Check sheet for the modelled part. Datum: model origin and axes. Units: mm. A direction names the side the tool comes from. Coordinates: 2 decimals unless noted, no trailing zeros. Write each loop counter-clockwise with the first axis right and the second up, starting at its lowest first coordinate (ties: lowest second). Pieces come first, ordered by that corner, then holes. Notation, with made-up numbers: (-13, 27.25) -> (39, 27.25) arc R31 cw to (39, 55.25) -> close; hole circle Ø1 at (57, 52). An arc over 180 degrees is marked (long way). Put each result on its own line as item: value.
```python
from build123d import *

# Parameters (mm, degrees)
SKETCH1_R           = 2.667
BOSS_EXTRUDE1_DEPTH = 4.7625
BOSS_EXTRUDE2_DEPTH = 50.8
SKETCH4_R           = 3.302
CUT_EXTRUDE1_DEPTH  = 55.626
BOSS_EXTRUDE3_DEPTH = 50.038
CUT_EXTRUDE5_DEPTH  = 46.0375
BOSS_EXTRUDE4_DEPTH = 3.175
BOSS_EXTRUDE5_DEPTH = 3.175
FILLET1_R           = 5.08
FILLET2_R           = 5.08


with BuildPart() as part:
    # Sketch1 → Boss-Extrude1 (new body)
    with BuildSketch(Plane(origin=(0, 0, 0), x_dir=(1, 0, 0), z_dir=(0, 1, 0))):
        Polygon((37.846, 50.038), (33.907923994, 0), (0, 0), (0, 50.038), align=None)
        with Locations(Location((12.7, 37.338, 0), (0, 0, 90))):
            Circle(SKETCH1_R, mode=Mode.SUBTRACT)
        with Locations(Location((25.4, 37.338, 0), (0, 0, 90))):
            Circle(SKETCH1_R, mode=Mode.SUBTRACT)
        with Locations(Location((12.7, 11.938, 0), (0, 0, 90))):
            Circle(SKETCH1_R, mode=Mode.SUBTRACT)
        with Locations(Location((25.4, 11.938, 0), (0, 0, 90))):
            Circle(SKETCH1_R, mode=Mode.SUBTRACT)
    extrude(amount=BOSS_EXTRUDE1_DEPTH)

    # Sketch2 → Boss-Extrude2 (add)
    with BuildSketch(Plane.XZ):
        Polygon((29.2288268, -1.246852262), (33.068773405, -50.038), (37.846, -50.038), (33.907923994, 0), (29.130697399, 0), (29.160105192, -0.373661443), align=None)
    extrude(amount=-BOSS_EXTRUDE2_DEPTH)

    # Sketch4 → Cut-Extrude1 (cut)
    with BuildSketch(Plane(origin=(28.951373786, 0, 2.278522532), x_dir=(-0.07845909572784877, 0, 0.9969173337331276), z_dir=(-0.9969173337331276, 0, -0.07845909572784877))):
        with Locations((-27.304568176, 25.4)):
            Circle(SKETCH4_R)
    extrude(amount=-CUT_EXTRUDE1_DEPTH, mode=Mode.SUBTRACT)

    # Sketch5 → Boss-Extrude3 (add)
    with BuildSketch(Plane.XY):
        Polygon((2.157923994, 4.7625), (33.907923994, 16.318554938), (33.907923994, 4.7625), align=None)
    extrude(amount=-BOSS_EXTRUDE3_DEPTH)

    # Sketch7 → Cut-Extrude5 (cut)
    with BuildSketch(Plane(origin=(0, 50.8, 0), x_dir=(1, 0, 0), z_dir=(0, 1, 0))):
        Polygon((33.068773405, 50.038), (31.224674361, 26.6065), (2.157923994, 26.6065), (2.157923994, 50.038), align=None)
        Polygon((2.157923994, 23.4315), (30.974796442, 23.4315), (29.130697399, 0), (2.157923994, 0), align=None)
    extrude(amount=-CUT_EXTRUDE5_DEPTH, mode=Mode.SUBTRACT)

    # Sketch8 → Boss-Extrude4 (add)
    with BuildSketch(Plane.XY):
        Polygon((2.157923994, 4.7625), (33.907923994, 49.2125), (33.907923994, 4.7625), align=None)
    extrude(amount=-BOSS_EXTRUDE4_DEPTH)

    # Sketch9 → Boss-Extrude5 (add)
    with BuildSketch(Plane(origin=(0, 0, -50.038), x_dir=(-1, 0, 0), z_dir=(0, 0, -1))):
        Polygon((-2.157923994, 4.7625), (-33.068773405, 47.9425), (-33.068773405, 4.7625), align=None)
    extrude(amount=-BOSS_EXTRUDE5_DEPTH)

    # Fillet1
    # the kernel refuses this fillet: 5.08 mm, written as the material it adds along each edge
    with BuildSketch(Plane(origin=(2.157923994, 4.7625, 0), x_dir=(-1, 0, 0), z_dir=(0, 0, -1))) as fillet1_piece_1:
        with BuildLine():
            CenterArc((2.629957643, 5.058021771), FILLET1_R, 215.537677792, 49.130706658)
            Line((-1.503808391, 2.105331747), (-1.586483711, 2.046277946))
            Line((-1.586483711, 2.046277946), (-0.082675321, -0.0590538))
            Line((-0.082675321, -0.0590538), (0, -0.1016))
            ThreePointArc((0, -0.1016), (1.078961997, -0.1016), (2.148483321, -0.101160435))
            Line((2.148483321, -0.101160435), (2.157923994, 0))
        make_face()
    extrude(amount=3.175)
    with BuildSketch(Plane(origin=(2.157923994, 4.7625, -50.038), x_dir=(-1, 0, 0), z_dir=(0, 0, 1))) as fillet1_piece_2:
        with BuildLine():
            CenterArc((2.626409807, -5.058351613), FILLET1_R, 95.291428018, 49.111198854)
            Line((-1.504277635, -2.101356304), (-1.586891383, -2.042216397))
            Line((-1.586891383, -2.042216397), (-0.082613749, 0.059139906))
            Line((-0.082613749, 0.059139906), (0, 0.1016))
            ThreePointArc((0, 0.1016), (1.078961997, 0.1016), (2.148554278, 0.101167032))
            Line((2.148554278, 0.101167032), (2.157923994, 0))
        make_face()
    extrude(amount=3.175)
    with BuildSketch(Plane(origin=(29.700338722, 43.32188062, -7.237979285), x_dir=(-0.008566636475351457, 0.9940213341844409, 0.10884943695620641), z_dir=(-0.07799001501429913, -0.10918602102001876, 0.9909570981489993))) as fillet1_piece_3_section:
        with BuildLine():
            CenterArc((FILLET1_R * 0.322839030398, FILLET1_R), FILLET1_R, 234.215790713, 35.784209287)
            Line((-FILLET1_R * 0.261895093237, FILLET1_R * 0.188774997515), (-FILLET1_R * 0.27358977571, FILLET1_R * 0.172550497465))
            Line((-FILLET1_R * 0.27358977571, FILLET1_R * 0.172550497465), (-FILLET1_R * 0.00645678060796, -FILLET1_R * 0.02))
            Line((-FILLET1_R * 0.00645678060796, -FILLET1_R * 0.02), (FILLET1_R * 0.322839030398, -FILLET1_R * 0.02))
            Line((FILLET1_R * 0.322839030398, -FILLET1_R * 0.02), (FILLET1_R * 0.322839030398, 0))
        make_face()
    fillet1_piece_3 = extrude(amount=11.404084587, mode=Mode.PRIVATE)
    fillet1_piece_3 = split(fillet1_piece_3, bisect_by=Plane(origin=(29.0621266, 42.760284123, 0), z_dir=(0, 0, -1)), keep=Keep.TOP, mode=Mode.PRIVATE)
    fillet1_piece_3 = split(fillet1_piece_3, bisect_by=Plane(origin=(29.0621266, 42.760284123, -3.175), z_dir=(0, 0, 1)), keep=Keep.TOP, mode=Mode.PRIVATE)
    add(fillet1_piece_3)
    with BuildSketch(Plane(origin=(32.498558986, 47.145955774, -42.792738849), x_dir=(-0.008548017001345628, 0.994047372778579, 0.1086128541073727), z_dir=(0.07799205797884924, 0.10894870661005905, -0.9909830564748416))) as fillet1_piece_4_section:
        with BuildLine():
            CenterArc((FILLET1_R * 0.32340916623, -FILLET1_R), FILLET1_R, 90, 35.843365579)
            Line((-FILLET1_R * 0.262162212759, -FILLET1_R * 0.189379151447), (-FILLET1_R * 0.273873640339, -FILLET1_R * 0.173166734476))
            Line((-FILLET1_R * 0.273873640339, -FILLET1_R * 0.173166734476), (-FILLET1_R * 0.0064681833246, FILLET1_R * 0.02))
            Line((-FILLET1_R * 0.0064681833246, FILLET1_R * 0.02), (FILLET1_R * 0.32340916623, FILLET1_R * 0.02))
            Line((FILLET1_R * 0.32340916623, FILLET1_R * 0.02), (FILLET1_R * 0.32340916623, 0))
        make_face()
    fillet1_piece_4 = extrude(amount=11.418482111, mode=Mode.PRIVATE)
    fillet1_piece_4 = split(fillet1_piece_4, bisect_by=Plane(origin=(32.749606974, 47.829296301, -50.038), z_dir=(0, 0, 1)), keep=Keep.TOP, mode=Mode.PRIVATE)
    fillet1_piece_4 = split(fillet1_piece_4, bisect_by=Plane(origin=(32.749606974, 47.829296301, -46.863), z_dir=(0, 0, -1)), keep=Keep.TOP, mode=Mode.PRIVATE)
    add(fillet1_piece_4)

    # Fillet2
    fillet2_edges = [part.edges().sort_by_distance(p)[0] for p in [
        (32.818895486, 27.004348608, -46.863),
        (29.380575318, 24.643299124, -3.175),
    ]]
    fillet(fillet2_edges, radius=FILLET2_R)


solid = part.part
```
Q1. Cross-section at A-A (x = 24). Record the cut outline in (y, z) (1 decimal).
Recorded:
outline: (0, -50) -> (35.3, -50) -> (35.3, -46.9) -> (4.8, -46.9) -> (4.8, -39.6) -> (0, -39.6) -> close; (0, -35.1) -> (4.8, -35.1) -> (4.8, -26.6) -> (12.7, -26.6) -> (12.7, -23.4) -> (4.8, -23.4) -> (4.8, -14.2) -> (0, -14.2) -> close; (0, -9.7) -> (4.8, -9.7) -> (4.8, -3.2) -> (35.3, -3.2) -> (35.3, 0) -> (0, 0) -> close
Q2. Depth check by flat-ended pin: P1, Ø6, axis at x = 22, z = -28, coming from the +Y side; P2, Ø5, axis at y = 17.5, z = -20.5, coming from the -X side; P3, Ø9.5, axis at x = 8.5, z = -23, coming from the +Y side. Enter the tip coordinate at first touch or a pass-through.
Recorded:
P1: stops at y = 12.95
P2: stops at x = 30.55
P3: stops at y = 8.79
Q3. Cross-section at C-C (y = 24.5). Record the cut outline in (x, z) (3 decimals).
Recorded:
outline: (16.256, -3.175) -> (24.685, -3.175) arc R5.08 cw to (29.749, -7.856) -> (30.844, -21.775) -> (35.592, -21.401) -> (33.908, 0) -> (16.256, 0) -> close; (16.287, -50.038) -> (37.846, -50.038) -> (36.091, -27.735) -> (31.343, -28.109) -> (32.388, -41.384) arc R5.08 cw to (27.323, -46.863) -> (16.287, -46.863) -> close
Q4. Cross-section at B-B (y = 4). Record the cut outline in (x, z) (3 decimals).
Recorded:
outline: (0, -50.038) -> (37.846, -50.038) -> (33.908, 0) -> (0, 0) -> close; hole circle Ø5.334 at (12.7, -37.338); hole circle Ø5.334 at (12.7, -11.938); hole circle Ø5.334 at (25.4, -37.338); hole circle Ø5.334 at (25.4, -11.938)
Q5. Cross-section at D-D (z = -20.5). Record the cut outline in (x, y).
Recorded:
outline: (0, 0) -> (35.52, 0) -> (35.52, 50.8) -> (30.74, 50.8) -> (30.74, 4.76) -> (0, 4.76) -> close
Q6. Tool access check on faces 4 (the flat face through (35.467, 25.044, -19.809)), 5 (the flat face through (23, 8, -26.606)). Record the directions out of +Z, -Z, +X, -X, +Y, -Y that give a thin tool (end or side, any length) a straight path to the whole face; none if there is none.
Recorded:
face 4: +Z, +X, +Y, -Y
face 5: -X, +Y
Q7. Material ranges on line 1 along Z through (x, y) = (12.7, 1.3) (3 decimals); line 2 along Z through (x, y) = (12, 2); line 3 along Z through (x, y) = (20, 18) (3 decimals), recorded low to high.
Recorded:
line 1: z = -50.038 to -40.005, -34.671 to -14.605, -9.271 to 0
line 2: z = -50.04 to -39.91, -34.76 to -14.51, -9.36 to 0
line 3: z = -50.038 to -46.863, -3.175 to 0
Q8. Mould release check, pull along X, two halves, no side actions. Record for faces 1 (the cylindrical face through (33.468, 28.674, -25.186)), 2 (the cylindrical face through (2.03, 5.4, -48.47)), 3 (the cylindrical face through (23.15, 2.35, -38.77)): released by +X, released by -X, zero draft, split by the parting line, or undercut.
Recorded:
face 1: split by the parting line
face 2: released by -X
face 3: undercut
